Design review of the part built by this model. Coordinates are the model's own, in mm. Face numbers are marked on the shaded views. A direction names the side the tool comes from. Round coordinates to 2 decimals unless told otherwise and drop trailing zeros. Order: outer loops, then holes, each group sorted by start corner. A loop starts at its lowest first (then second) coordinate and runs counter-clockwise, first axis right, second up.
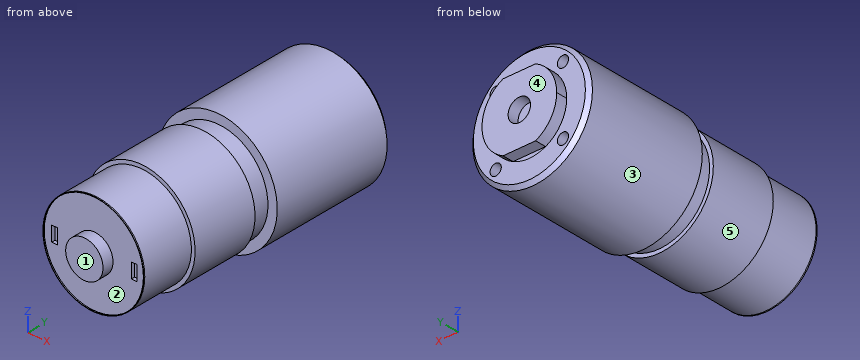
Autodesk Inventor part; units mm, degrees
ref_plane "YZ Plane" through (0, 0, 0) normal (1, 0, 0) x (0, 1, 0)
ref_plane "XZ Plane" through (0, 0, 0) normal (0, 1, 0) x (-1, 0, 0)
ref_plane "XY Plane" through (0, 0, 0) normal (0, 0, 1) x (1, 0, 0)
sketch "スケッチ1" plane through (0, 0, 0) normal (0, 0, 1) x (1, 0, 0)
  line L0 (0, 0) -> (-16, 0)
  line L1 (-16, 0) -> (-16, 34)
  line L2 (-16, 34) -> (0, 34)
  line L3 (0, 34) -> (0, 0)
  line L4 (0, 34) -> (-10, 34)
  line L5 (-10, 34) -> (-10, 37)
  line L6 (-10, 37) -> (0, 37)
  line L7 (0, 37) -> (0, 34)
  line L8 (0, 37) -> (-5, 37)
  line L9 (-5, 34) -> (0, 34)
  line L10 (0, 34) -> (0, 37)
  line L11 (-3, 37) -> (-3, 34)
  line L12 (-13.5, 0) -> (0, 0)
  line L13 (0, 0) -> (0, -37)
  line L14 (0, -37) -> (-13.5, -37)
  line L15 (-13.5, -37) -> (-13.5, 0)
  line L16 (-13.5, 0) -> (-14.5, 0)
  line L17 (-13.5, -23) -> (-13.5, 0)
  line L18 (-13.5, -5) -> (-14.5, -5)
  line L19 (-14.5, -5) -> (-14.5, -23)
  line L20 (-14.5, -23) -> (-13.5, -23)
  line L21 (-13.5, -23) -> (-13.5, -5)
  line L22 (0, -37) -> (-5, -37)
  line L23 (-5, -37) -> (-5, -40)
  line L24 (-5, -40) -> (0, -40)
  line L25 (0, -40) -> (0, -37)
  dimension "d0" = 16
  dimension "d1" = 34
  dimension "d2" = 10
  dimension "d4" = 3
  dimension "d5" = 3
  dimension "d6" = 13.5
  dimension "d7" = 0
  dimension "d10" = 37
  dimension "d11" = 5
  dimension "d12" = 14
  dimension "d13" = 1
  dimension "d14" = 3
  dimension "d15" = 5
revolve "回転1" add sketch "スケッチ1" angle 360 about axis through (0, 34, 0) along (0, -1, 0) contours L13 L14 L15 L0 | L0 L1 L2 L3 | L25 L24 L23 L14 | L15 L20 L19 L18 | L2 L5 L6 L11
chamfer "面取り1" distance 1 angle 45 1 edges at (16, 34, 0)
sketch "スケッチ2" plane through (0, -37, 0) normal (0, -1, 0) x (1, 0, 0)
  circle A0 centre (0, 0) radius 5
  circle A1 centre (0, 0) radius 13.4
  circle A2 centre (0, 0) radius 13.5
  circle A3 centre (0, 0) radius 13.5
  line L0 (-9.9, -2) -> (-11.4, -2)
  line L1 (-11.4, -2) -> (-11.4, 2)
  line L2 (-11.4, 2) -> (-9.9, 2)
  line L3 (-9.9, 2) -> (-9.9, -2)
  line L4 (-9.9, -2) -> (-11.4, 2) construction
  line L5 (-11.4, -2) -> (-9.9, 2) construction
  line L6 (11.4, -2) -> (9.9, -2)
  line L7 (9.9, -2) -> (9.9, 2)
  line L8 (9.9, 2) -> (11.4, 2)
  line L9 (11.4, 2) -> (11.4, -2)
  line L10 (11.4, -2) -> (9.9, 2) construction
  line L11 (9.9, -2) -> (11.4, 2) construction
  line L12 (-13.4, 0) -> (0, 0)
  line L13 (0, 0) -> (13.4, 0)
  point P0 (-10.65, 0)
  point P1 (10.65, 0)
  dimension "d21" = 0
  dimension "d22" = 0.1
  dimension "d23" = 1.5
  dimension "d24" = 1.5
  dimension "d25" = 4
  dimension "d26" = 4
  dimension "d27" = 0
  dimension "d28" = 2
  dimension "d29" = 2
extrude "押し出し1" add sketch "スケッチ2" along normal blind 0.3
extrude "押し出し2" cut sketch "スケッチ2" against normal blind 1 contours L13 L9 L6 L7 | L7 L8 L9 L13 | L12 L1 L2 L3 | L3 L0 L1 L12
sketch "スケッチ3" plane through (0, 34, 0) normal (0, 1, 0) x (1, 0, 0)
  circle A0 centre (0, 0) radius 15
  circle A1 centre (-9, -9) radius 1.5
  circle A2 centre (-9, 9) radius 1.5
  circle A3 centre (9, 9) radius 1.5
  circle A4 centre (9, -9) radius 1.5
  line L0 (9, -9) -> (-9, -9)
  line L1 (-9, -9) -> (-9, 9)
  point P0 (0, 0)
  dimension "d54" = 18
  dimension "d55" = 18
  dimension "d56" = 18
  dimension "d57" = 18
  dimension "d58" = 0
  dimension "d59" = 3
  dimension "d60" = 3
  dimension "d61" = 3
  dimension "d62" = 3
  dimension "d63" = 9
  dimension "d64" = 9
extrude "押し出し5" cut sketch "スケッチ3" against normal blind 9.5 contours L0 L1 A1 | A2 | A1 L1 L0 | A4 | A3
sketch "スケッチ6" plane through (0, 37, 0) normal (0, 1, 0) x (1, 0, 0)
  circle A0 centre (0, 0) radius 10
  line L0 (-4.3589, -9) -> (4.3589, -9)
  line L1 (-4.3589, 9) -> (4.3589, 9)
  line L2 (0, 10) -> (0, 9)
  line L3 (0, -9) -> (0, -10)
  arc A1 (-4.3589, -9) -> (4.3589, -9) centre (0, 0) ccw
  arc A2 (4.3589, 9) -> (-4.3589, 9) centre (0, 0) ccw
  point P0 (0, 0)
  dimension "d67" = 1
  dimension "d68" = 1
extrude "押し出し6" cut sketch "スケッチ6" against normal blind 3 contours L1 L2 A0 | A0 L3 L0 | L2 L1 A0 | A0 L0 L3
properties part number "モーター100：1"
1) Take a section at B-B on y = -21. Give the boundary of the cut face in (x, z).
Results:
outline: circle Ø29 at (0, 0)
2) To check wall thickness, follow line 1 along Z through (x, y) = (10, 29.5); line 2 along Z through (x, y) = (-9, 31.75). State the ranges of each line that lie inside material, in increasing order.
Results:
line 1: z = -12.49 to -10.12, -7.88 to 7.88, 10.12 to 12.49
line 2: z = -13.23 to -10.5, -7.5 to 7.5, 10.5 to 13.23
3) Clearance check with flat-ended pins moving along their axes: P1, Ø4, axis at x = 9, z = 9, coming from the +Y side; P2, Ø5, axis at y = 16.5, z = -8, coming from the +X side (3 decimals); P3, Ø2, axis at x = 12, y = -15, coming from the +Z side. State where each tip first meets the part, or that it passes through.
Results:
P1: stops at y = 34
P2: stops at x = 15.025
P3: stops at z = 9.45
4) Take a section at C-C on y = 12. Give the boundary of the cut face in (x, z).
Results:
outline: circle Ø32 at (0, 0)
5) For the marked faces 4 and 5, list the 3-axis set-ups (+Z, -Z, +X, -X, +Y, -Y) from which the entire face can be reached by the end or side of a thin tool; tool diameter is ignored.
Results:
face 4: +Z, -Z, +X, -X, +Y
face 5: -Y
6) The part is to be moulded in two halves that separate along Z. For the marked faces 1, 2 and 3, say which applies: released by +Z, released by -Z, zero draft, split by the parting line, or undercut.
Results:
face 1: zero draft
face 2: undercut
face 3: split by the parting line
